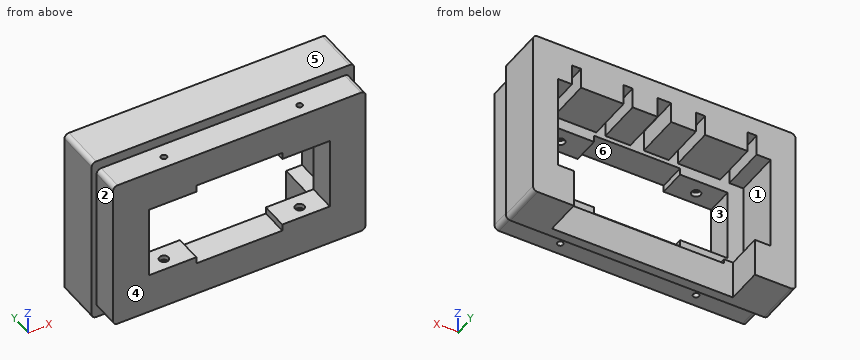
from build123d import *

# Parameters (mm, degrees)
SKETCH1_W               = 279
SKETCH1_H               = 169
BOSS_EXTRUDE1_DEPTH     = 30
SKETCH2_W               = 290
SKETCH2_H               = 190
BOSS_EXTRUDE2_DEPTH     = 50
FILLET1_R               = 5
FILLET2_R               = 5
SKETCH3_W               = 235
SKETCH3_H               = 105
CUT_EXTRUDE1_DEPTH      = 50
SKETCH4_W               = 200
SKETCH4_H               = 80
CUT_EXTRUDE2_DEPTH      = 50
SKETCH5_W               = 180
SKETCH5_H               = 5
CUT_EXTRUDE3_DEPTH      = 50
SKETCH6_W               = 95
SKETCH6_H               = 95
CUT_EXTRUDE4_DEPTH      = 50
SKETCH7_W               = 15
SKETCH7_H               = 23
SKETCH7_W_2             = 10
CUT_EXTRUDE5_DEPTH      = 50
SKETCH8_R               = 3.25
CUT_EXTRUDE6_DEPTH      = 180.5
SKETCH9_R               = 5
CUT_EXTRUDE7_DEPTH      = 45
CUT_EXTRUDE7_DEPTH_BACK = 45
SKETCH11_W              = 200
SKETCH11_H              = 40
CUT_EXTRUDE9_DEPTH      = 50


with BuildPart() as part:
    # Sketch1 → Boss-Extrude1 (new body)
    with BuildSketch(Plane(origin=(0, 0, 0), x_dir=(1, 0, 0), z_dir=(0, 1, 0))):
        Rectangle(SKETCH1_W, SKETCH1_H)
    extrude(amount=-BOSS_EXTRUDE1_DEPTH)

    # Sketch2 → Boss-Extrude2 (add)
    with BuildSketch(Plane(origin=(0, 0, 0), x_dir=(1, 0, 0), z_dir=(0, 1, 0))):
        Rectangle(SKETCH2_W, SKETCH2_H)
    extrude(amount=BOSS_EXTRUDE2_DEPTH)

    # Fillet1
    fillet1_edges = [part.edges().sort_by_distance(p)[0] for p in [
        (139.5, -15, 84.5),
        (-139.5, -15, 84.5),
        (-139.5, -15, -84.5),
        (139.5, -15, -84.5),
    ]]
    fillet(fillet1_edges, radius=FILLET1_R)

    # Fillet2
    fillet2_edges = [part.edges().sort_by_distance(p)[0] for p in [
        (145, 25, 95),
        (145, 25, -95),
        (-145, 25, -95),
        (-145, 25, 95),
    ]]
    fillet(fillet2_edges, radius=FILLET2_R)

    # Sketch3 → Cut-Extrude1 (cut)
    with BuildSketch(Plane(origin=(0, 50, 0), x_dir=(1, 0, 0), z_dir=(0, 1, 0))):
        Rectangle(SKETCH3_W, SKETCH3_H)
    extrude(amount=-CUT_EXTRUDE1_DEPTH, mode=Mode.SUBTRACT)

    # Sketch4 → Cut-Extrude2 (cut)
    with BuildSketch(Plane(origin=(0, 0, 0), x_dir=(1, 0, 0), z_dir=(0, 1, 0))):
        Rectangle(SKETCH4_W, SKETCH4_H)
    extrude(amount=-CUT_EXTRUDE2_DEPTH, mode=Mode.SUBTRACT)

    # Sketch5 → Cut-Extrude3 (cut)
    with BuildSketch(Plane(origin=(0, 50, 0), x_dir=(1, 0, 0), z_dir=(0, 1, 0))):
        with Locations((0, 55)):
            Rectangle(SKETCH5_W, SKETCH5_H)
    extrude(amount=-CUT_EXTRUDE3_DEPTH, mode=Mode.SUBTRACT)

    # Sketch6 → Cut-Extrude4 (cut)
    with BuildSketch(Plane(origin=(0, 0, 0), x_dir=(1, 0, 0), z_dir=(0, 1, 0))):
        Rectangle(SKETCH6_W, SKETCH6_H)
    extrude(amount=-CUT_EXTRUDE4_DEPTH, mode=Mode.SUBTRACT)

    # Sketch7 → Cut-Extrude5 (cut)
    with BuildSketch(Plane(origin=(0, 50, 0), x_dir=(1, 0, 0), z_dir=(0, 1, 0))):
        with Locations((0, -64)):
            Rectangle(SKETCH7_W, SKETCH7_H)
        with Locations((40, -64)):
            Rectangle(SKETCH7_W_2, SKETCH7_H)
        with Locations((-40, -64)):
            Rectangle(SKETCH7_W_2, SKETCH7_H)
        with Locations((97, -64)):
            Rectangle(SKETCH7_W_2, SKETCH7_H)
        with Locations((-97, -64)):
            Rectangle(SKETCH7_W_2, SKETCH7_H)
    extrude(amount=-CUT_EXTRUDE5_DEPTH, mode=Mode.SUBTRACT)

    # Sketch8 → Cut-Extrude6 (cut, through all)
    with BuildSketch(Plane(origin=(0, 0, -84.5), x_dir=(-1, 0, 0), z_dir=(0, 0, -1))):
        with Locations((75, -16.25)):
            Circle(SKETCH8_R)
        with Locations((-75, -16.25)):
            Circle(SKETCH8_R)
    extrude(amount=-CUT_EXTRUDE6_DEPTH, mode=Mode.SUBTRACT)

    # Sketch9 → Cut-Extrude7 (cut, two sides)
    with BuildSketch(Plane.XY) as cut_extrude7_sk:
        with Locations((-75, -16.25)):
            Circle(SKETCH9_R)
        with Locations((75, -16.25)):
            Circle(SKETCH9_R)
    extrude(amount=CUT_EXTRUDE7_DEPTH, mode=Mode.SUBTRACT)
    extrude(cut_extrude7_sk.sketch, amount=-CUT_EXTRUDE7_DEPTH_BACK, mode=Mode.SUBTRACT)

    # Sketch11 → Cut-Extrude9 (cut)
    with BuildSketch(Plane(origin=(0, 0, -95), x_dir=(-1, 0, 0), z_dir=(0, 0, -1))):
        with Locations((0, 30)):
            Rectangle(SKETCH11_W, SKETCH11_H)
    extrude(amount=-CUT_EXTRUDE9_DEPTH, mode=Mode.SUBTRACT)


solid = part.part
Build history of the part. All positions in model axes, mm. Face numbers are marked on the shaded views. A direction names the side the tool comes from. Round coordinates to 2 decimals unless told otherwise and drop trailing zeros. Write each loop counter-clockwise with the first axis right and the second up, starting at its lowest first coordinate (ties: lowest second). Pieces come first, ordered by that corner, then holes. Notation, with made-up numbers: (-20, 8.5) -> (13, 8.5) arc R19 ccw to (13, 27.5) -> close; hole circle Ø4 at (11, 78). An arc over 180 degrees is marked (long way). Use one line per item in the form item = value.
Q1. Drill centre lines: L1, parallel to X at y = 1.5, z = 63; L2, parallel to X at y = -16, z = -68; L3, parallel to X at y = 8, z = -1.5. Where is each one in solid material? Low to high.
Conclusion:
L1 = -145 to -102, -92 to -45, -35 to -7.5, 7.5 to 35, 45 to 92, 102 to 145
L2 = -139.5 to -78.24, -71.76 to 71.76, 78.24 to 139.5
L3 = -145 to -117.5, 117.5 to 145
Q2. Band-saw the part on A-A, the plane x = 64. Write the cut outline in (y, z), then the cut area to 3 significant figures.
Conclusion:
outline = (-30, -84.5) -> (0, -84.5) -> (0, -95) -> (10, -95) -> (10, -57.5) -> (0, -57.5) -> (0, -40) -> (-30, -40) -> close; (-30, 40) -> (0, 40) -> (0, 52.5) -> (50, 52.5) -> (50, 95) -> (0, 95) -> (0, 84.5) -> (-30, 84.5) -> close
area = 5,170 mm²
Q3. Two-plate mould, pull along Z, no slides. Class the marked faces 4, 5 and 6: released by +Z, released by -Z, zero draft, split by the parting line, or undercut.
Conclusion:
face_4 = zero draft
face_5 = released by +Z
face_6 = undercut
Q4. Band-saw the part on B-B, the plane z = -1.5. Write the cut outline in (x, y), then the cut area to 3 significant figures.
Conclusion:
outline = (-145, 0) -> (-139.5, 0) -> (-139.5, -30) -> (-100, -30) -> (-100, 0) -> (-117.5, 0) -> (-117.5, 50) -> (-145, 50) -> close; (100, -30) -> (139.5, -30) -> (139.5, 0) -> (145, 0) -> (145, 50) -> (117.5, 50) -> (117.5, 0) -> (100, 0) -> close
area = 5,120 mm²
Q5. Band-saw the part on D-D, the plane y = -16.25. State how many separate pieces and enclosed holes the cut face has, then the cut area to 3 significant figures.
Conclusion:
separate_pieces = 4
enclosed_holes = 0
area = 28,500 mm²
Q6. Tool access for the marked faces 1, 2 and 3: list every direction of +Z, -Z, +X, -X, +Y, -Y with a clear straight run to the whole face (end or side of a thin tool).
Conclusion:
face_1 = +Y
face_2 = +Z, -Z, -X, -Y
face_3 = +Y, -Y
Q7. Drop flat-ended pins along their axis: P1, Ø8, axis at x = 39.5, y = 19.5, coming from the -Z side; P2, Ø3, axis at x = -57, y = 33, coming from the -Z side; P3, Ø24, axis at x = 20, y = -20.5, coming from the +Z side. Give the stop position or say it passes through.
Conclusion:
P1 = 75.5
P2 = 52.5
P3 = 84.5
Q8. Band-saw the part on C-C, the plane x = -112.5. Write the cut outline in (y, z), then the cut area to 3 significant figures.
Conclusion:
outline = (-30, -84.5) -> (0, -84.5) -> (0, -95) -> (50, -95) -> (50, -52.5) -> (0, -52.5) -> (0, 52.5) -> (50, 52.5) -> (50, 95) -> (0, 95) -> (0, 84.5) -> (-30, 84.5) -> close
area = 9,320 mm²
